Geometry check sheet. Reference: the model listing, model coordinates, mm. A direction names the side the tool comes from. Give positions to 0.01 mm unless a question says otherwise; leave off trailing zeros. Loops run counter-clockwise (first coordinate to the right, second up) from the corner with the lowest first, then second, coordinate; pieces in that order, holes last. Notation, with made-up numbers: (64.25, 65.25) -> (80.25, 65.25) arc R18 cw to (80.25, 98.25) -> close; hole circle Ø10 at (65, 65.25). An arc over 180 degrees is marked (long way). One line per question, with ' | ' between items.
from build123d import *

# Parameters (mm, degrees)
SKETCH020_R             = 8.5
SKETCH020_W             = 4.82
SKETCH020_H             = 2.55
PAD013_DEPTH            = 10
SKETCH021_R             = 7.75
SKETCH021_R_2           = 6.75
POCKET010_DEPTH         = 5
SKETCH022_R             = 5.45
POCKET011_DEPTH         = 5
SKETCH023_R             = 3.25
POCKET012_DEPTH         = 2
BODY006_PLACEMENT_ANGLE = 270


with BuildPart() as part:
    # Sketch020 → Pad013 (new body)
    with BuildSketch(Plane.XY):
        Circle(SKETCH020_R)
        Rectangle(SKETCH020_W, SKETCH020_H, mode=Mode.SUBTRACT)
    extrude(amount=PAD013_DEPTH)

    # Sketch021 (on Face7 of Pad013) → Pocket010 (cut)
    with BuildSketch(Plane.XY.offset(10)):
        Circle(SKETCH021_R)
        Circle(SKETCH021_R_2, mode=Mode.SUBTRACT)
    extrude(amount=-POCKET010_DEPTH, mode=Mode.SUBTRACT)

    # Sketch022 (on Face9 of Pocket010) → Pocket011 (cut)
    with BuildSketch(Plane.XY.offset(10)):
        Circle(SKETCH022_R)
    extrude(amount=-POCKET011_DEPTH, mode=Mode.SUBTRACT)

    # Sketch023 (on Face9 of Pocket011) → Pocket012 (cut)
    with BuildSketch(Plane.XY.offset(5)):
        Circle(SKETCH023_R)
    extrude(amount=-POCKET012_DEPTH, mode=Mode.SUBTRACT)


with BuildPart() as part_1:
    # Body006 placement: moved
    add(part.part.moved(Location((41.45, -89.75, 15.2))).rotate(Axis((41.45, -89.75, 15.2), (1, 0, 0)), BODY006_PLACEMENT_ANGLE))


solid = part_1.part
Item 1: Sectioned sample at D-D (y = -88). Record the cut outline in (x, z) (3 decimals), plus the area to 3 significant figures.
Result:
outline: circle Ø17 at (41.45, 15.2); hole (39.04, 13.925) -> (43.86, 13.925) -> (43.86, 16.475) -> (39.04, 16.475) -> close | area: 215 mm2
Item 2: Scan lines: probe 1 along Z at (x, y) = (41.45, -81.8); probe 2 along Z at (x, y) = (39.5, -80.5); probe 3 along X at (y, z) = (-83, 12.75). Record each from-to range of solid material in increasing order.
Result:
probe 1: 6.7 to 7.45, 8.45 to 9.75, 20.65 to 21.95, 22.95 to 23.7 | probe 2: 6.93 to 7.7, 8.74 to 10.11, 20.29 to 21.66, 22.7 to 23.47 | probe 3: 33.31 to 34.1, 35.16 to 36.58, 46.32 to 47.74, 48.8 to 49.59
Item 3: Sectioned sample at C-C (y = -81.5). Record the cut outline in (x, z).
Result:
outline: circle Ø17 at (41.45, 15.2); circle Ø13.5 at (41.45, 15.2); hole circle Ø15.5 at (41.45, 15.2); hole circle Ø10.9 at (41.45, 15.2)
Item 4: Sectioned sample at A-A (x = 41.45). Record the cut outline in (y, z) (3 decimals), plus the area to 4 significant figures.
Result:
outline: (-89.75, 6.7) -> (-79.75, 6.7) -> (-79.75, 7.45) -> (-84.75, 7.45) -> (-84.75, 8.45) -> (-79.75, 8.45) -> (-79.75, 9.75) -> (-84.75, 9.75) -> (-84.75, 11.95) -> (-86.75, 11.95) -> (-86.75, 13.925) -> (-89.75, 13.925) -> close; (-89.75, 16.475) -> (-86.75, 16.475) -> (-86.75, 18.45) -> (-84.75, 18.45) -> (-84.75, 20.65) -> (-79.75, 20.65) -> (-79.75, 21.95) -> (-84.75, 21.95) -> (-84.75, 22.95) -> (-79.75, 22.95) -> (-79.75, 23.7) -> (-89.75, 23.7) -> close | area: 84.85 mm2
Item 5: Set-up check for faces 4 (the face through (41, -88, 16.475)), 5 (the face through (38.2, -85.7, 15.1)), 6 (the face through (47, -79.75, 16)): record each of +Z, -Z, +X, -X, +Y, -Y from which the full face is reachable in a straight line by a thin tool's end or side.
Result:
face 4: +Y, -Y | face 5: +Y | face 6: +Z, -Z, +X, -X, +Y
Item 6: Depth check by flat-ended pin: pin 1 Ø2 at (y, z) = (-88, 15.5) entering from -X; pin 2 Ø3 at (x, z) = (40, 14.5) entering from +Y; pin 3 Ø1.5 at (x, y) = (42.5, -88.5) entering from +Z; pin 4 Ø1 at (y, z) = (-87, 9) entering from -X. Enter the tip coordinate at first touch or a pass-through.
Result:
pin 1: x = 32.95 | pin 2: y = -86.75 | pin 3: z = 23.69 | pin 4: x = 35.14
Item 7: Sectioned sample at B-B (z = 15.2). Record the cut outline in (x, y), plus the area to 3 significant figures.
Result:
outline: (32.95, -89.75) -> (39.04, -89.75) -> (39.04, -86.75) -> (38.2, -86.75) -> (38.2, -84.75) -> (36, -84.75) -> (36, -79.75) -> (34.7, -79.75) -> (34.7, -84.75) -> (33.7, -84.75) -> (33.7, -79.75) -> (32.95, -79.75) -> close; (43.86, -89.75) -> (49.95, -89.75) -> (49.95, -79.75) -> (49.2, -79.75) -> (49.2, -84.75) -> (48.2, -84.75) -> (48.2, -79.75) -> (46.9, -79.75) -> (46.9, -84.75) -> (44.7, -84.75) -> (44.7, -86.75) -> (43.86, -86.75) -> close | area: 78.0 mm2
Item 8: Release check for a two-part mould opening along X. For faces 1 (the face through (39.04, -88, 15)), 2 (the face through (40, -79.75, 23)), 3 (the face through (35.185, -84.82, 9.455)) record: pulls with the +X half, pulls with the -X half, needs draft (parallel to the pull), parting line crosses it, or undercut.
Result:
face 1: undercut | face 2: needs draft | face 3: parting line crosses it
